Build history of the part. All positions in model axes, mm. Face numbers are marked on the shaded views. A direction names the side the tool comes from. Give positions to 0.01 mm unless a question says otherwise; leave off trailing zeros. Write each loop counter-clockwise with the first axis right and the second up, starting at its lowest first coordinate (ties: lowest second). Pieces come first, ordered by that corner, then holes. Notation, with made-up numbers: (8, -37) -> (31, -37) arc R16 ccw to (31, -8) -> close; hole circle Ø10 at (48, -31.5). An arc over 180 degrees is marked (long way). Put each result on its own line as item: value. Start each with the question number.
Item 1: Tool access for the marked faces 5, 6 and 7: list every direction of +Z, -Z, +X, -X, +Y, -Y with a clear straight run to the whole face (end or side of a thin tool).
Item 2: Slice it at D-D, the plane z = 1.2. List the corners of the cut face in (x, y), plus the area to 3 significant figures.
Item 3: Slice it at B-B, the plane y = 0. List the corners of the cut face in (x, z) (3 decimals).
Item 4: Slice it at A-A, the plane z = 0. List the corners of the cut face in (x, y) (3 decimals), plus the area to 3 significant figures.
Item 5: Drill centre lines: line 1 along X through (y, z) = (-5.75, 0); line 2 along Y through (x, z) = (0, -1.85); line 3 along Z through (x, y) = (-1.5, -4). Where is each one in solid material? Low to high.
Item 6: Two-plate mould, pull along X, no slides. Class the marked faces 1, 2, 3 and 4: pulls with the +X half, pulls with the -X half, needs draft (parallel to the pull), parting line crosses it, or undercut.
Item 7: Flat gauge pins, fed straight in: pin 1 Ø3 at (x, y) = (1.5, -5) entering from +Z; pin 2 Ø2.5 at (x, z) = (0.5, 0) entering from -Y; pin 3 Ø1 at (x, z) = (2.5, 1.5) entering from +Y; pin 4 Ø2 at (x, y) = (-1, -6) entering from -Z. Where does each tip first touch, or does it go through?
Item 8: Slice it at C-C, the plane x = 0. List the corners of the cut face in (y, z) (3 decimals).
```python
from build123d import *

# Parameters (mm, degrees)
SOCKET_OUTER_EYE_AND_MOUTHS_START              = -2.2
SKETCH1_R                                      = 3.5
SKETCH1_R_2                                    = 2.2
SOCKET_OUTER_EYE_AND_MOUTHS_DEPTH              = 4.4
ROD_CONNECTION_NECK_START                      = -2
SKETCH2_W                                      = 4
SKETCH2_H                                      = 5.3
ROD_CONNECTION_NECK_DEPTH                      = 4
SKETCH3_R                                      = 1.05
D2P1_ROD_BOND_BORE_DEPTH                       = 2.7
SKETCH4_R                                      = 3
REVB_M6X0P35_CAP_FEMALE_THREAD_MAJOR_POC_DEPTH = 1.4


# Read off the part's stored shape, not the designer's step: Spherical_Socket_D5p05
with BuildPart() as part:
    # Sketch1 → Socket_Outer_Eye_And_Mouths (new body)
    with BuildSketch(Plane.XY.offset(SOCKET_OUTER_EYE_AND_MOUTHS_START)):
        Circle(SKETCH1_R)
        Circle(SKETCH1_R_2, mode=Mode.SUBTRACT)
    extrude(amount=SOCKET_OUTER_EYE_AND_MOUTHS_DEPTH)

    # Sketch2 → Rod_Connection_Neck (add)
    with BuildSketch(Plane.XY.offset(ROD_CONNECTION_NECK_START)):
        with Locations((0, -4.85)):
            Rectangle(SKETCH2_W, SKETCH2_H)
    extrude(amount=ROD_CONNECTION_NECK_DEPTH)

    # Spherical_Socket_D5p05 outline → Spherical_Socket_D5p05 (revolve, cut)
    with BuildSketch(Plane.XZ):
        with BuildLine():
            Line((2.199999999, 1.239203375), (2.199999999, -1.239203375))
            ThreePointArc((2.199999999, -1.239203375), (2.525, 0), (2.199999999, 1.239203375))
        make_face()
    revolve(axis=Axis((0, 0, 0), (0, 0, 1)), mode=Mode.SUBTRACT)

    # Sketch3 → D2p1_Rod_Bond_Bore (cut)
    with BuildSketch(Plane.XZ.offset(7.5)):
        with Locations(Location((0, 0, 0), (0, 0, 270))):
            Circle(SKETCH3_R)
    extrude(amount=-D2P1_ROD_BOND_BORE_DEPTH, mode=Mode.SUBTRACT)

    # Sketch4 → RevB_M6x0p35_Cap_Female_Thread_Major_Pocket (cut)
    with BuildSketch(Plane.XY.offset(2.2)):
        Circle(SKETCH4_R)
    extrude(amount=-REVB_M6X0P35_CAP_FEMALE_THREAD_MAJOR_POC_DEPTH, mode=Mode.SUBTRACT)


solid = part.part
```
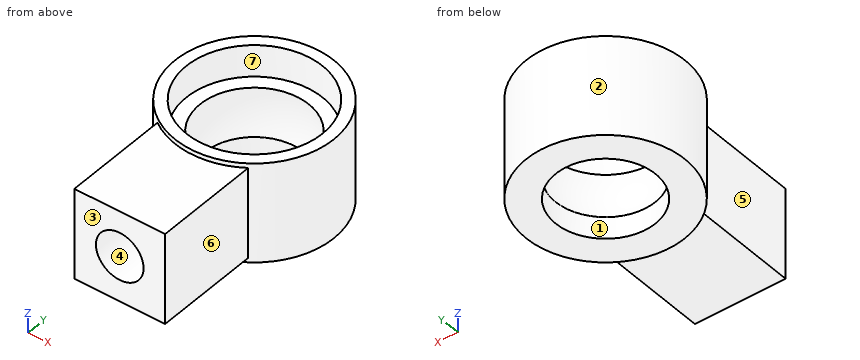
Values follow:
1. face 5: +Z, -Z, -X, -Y
1. face 6: +Z, -Z, +X, -Y
1. face 7: +Z
2. outline: (-2, -7.5) -> (2, -7.5) -> (2, -2.87) arc R3.5 ccw (long way) to (-2, -2.87) -> close; hole circle Ø6 at (0, 0)
2. area: 27.0 mm2
3. outline: (-3.5, -2.2) -> (-2.2, -2.2) -> (-2.2, -1.239) arc R2.525 cw to (-2.395, 0.8) -> (-3, 0.8) -> (-3, 2.2) -> (-3.5, 2.2) -> close; (2.2, -2.2) -> (3.5, -2.2) -> (3.5, 2.2) -> (3, 2.2) -> (3, 0.8) -> (2.395, 0.8) arc R2.525 cw to (2.2, -1.239) -> close
4. outline: (-2, -7.5) -> (-1.05, -7.5) -> (-1.05, -4.8) -> (1.05, -4.8) -> (1.05, -7.5) -> (2, -7.5) -> (2, -2.872) arc R3.5 ccw (long way) to (-2, -2.872) -> close; hole circle Ø5.05 at (0, 0)
4. area: 29.6 mm2
5. line 1: -2 to -1.05, 1.05 to 2
5. line 2: -7.5 to -2.2, 2.2 to 3.5
5. line 3: -2 to 2
6. face 1: undercut
6. face 2: parting line crosses it
6. face 3: needs draft
6. face 4: undercut
7. pin 1: z = 2
7. pin 2: y = -7.5
7. pin 3: y = 2.87
7. pin 4: z = -2
8. outline: (-7.5, -2) -> (-3.5, -2) -> (-3.5, -2.2) -> (-2.2, -2.2) -> (-2.2, -1.239) arc R2.525 cw to (-2.395, 0.8) -> (-3, 0.8) -> (-3, 2.2) -> (-3.5, 2.2) -> (-3.5, 2) -> (-7.5, 2) -> (-7.5, 1.05) -> (-4.8, 1.05) -> (-4.8, -1.05) -> (-7.5, -1.05) -> close; (2.2, -2.2) -> (3.5, -2.2) -> (3.5, 2.2) -> (3, 2.2) -> (3, 0.8) -> (2.395, 0.8) arc R2.525 cw to (2.2, -1.239) -> close
